Read the model definition and answer for the solid it produces. Units are mm, in the model's axes. A direction names the side the tool comes from. Coordinates: 2 decimals unless noted, no trailing zeros. Loops run counter-clockwise (first coordinate to the right, second up) from the corner with the lowest first, then second, coordinate; pieces in that order, holes last. Notation, with made-up numbers: M 74,-16 L 108,-16 A12 ccw 108,-10 Z; hole C 6,30.5 d6. An arc over 180 degrees is marked long. One line per item, written item: value. Start each with the question number.
1. Determine the mould class of faces 1 (the face through (-34.889, 25, 9)), 2 (the face through (-20.76, 42.07, 0.9)), 3 (the face through (-15, 25, 30.95)) for opening direction X: +X half, -X half, draft (parallel to the pull), parting line (faces both ways), or undercut.
2. The part is cut by section C-C (y = 10.5). Write down the section's boundary in (x, z), then the cut area to 3 significant figures.
3. The part is cut by section B-B (x = -6). Write down the section's boundary in (y, z), then the cut area to 3 significant figures.
4. For faces 4 (the face through (-32.889, 14, 9)), 5 (the face through (-14, 2, 8)), 6 (the face through (-23, 47, 15)), determine the directions among +Z, -Z, +X, -X, +Y, -Y from which every point of the face is accessible in a straight line to the end or side of a thin tool.
5. Flat-ended cylindrical pins translate along their axes: pin 1 (11.5 mm diameter, centred on x = -10, z = 16, fed in from +Y); pin 2 (16 mm diameter, centred on x = -22.5, z = 11, fed in from +Y); pin 3 (2 mm diameter, centred on x = 4.5, z = 14, fed in from -Y). Find the tip coordinate at first contact, or state that the pin passes through.
6. Consider probe 1 along Z at (x, y) = (-24, 10.5); probe 2 along Y at (x, z) = (-31, -1.5); probe 3 along X at (y, z) = (41, -8.5). Determine where each line is inside the solid, lowest interval first.
7. The part is cut by section D-D (y = 45). Write down the section's boundary in (x, z).
8. The part is cut by section A-A (z = 23.5). Write down the section's boundary in (x, y), then the cut area to 3 significant figures.
```python
from build123d import *

# Parameters (mm, degrees)
SKETCH1_W           = 40
SKETCH1_H           = 45
BOSS_EXTRUDE1_DEPTH = 50
SHELL1_T            = -2
SKETCH2_W           = 41
SKETCH2_H           = 15
CUT_EXTRUDE1_DEPTH  = 3
SKETCH4_W           = 41
SKETCH4_H           = 10
BOSS_EXTRUDE2_DEPTH = 20
SKETCH17_R          = 2.5
BOSS_EXTRUDE3_DEPTH = 10
BOSS_EXTRUDE3_TAPER = 3
SKETCH16_R          = 2.5
BOSS_EXTRUDE4_DEPTH = 10
BOSS_EXTRUDE4_TAPER = 3


with BuildPart() as part:
    # Sketch1 → Boss-Extrude1 (new body)
    with BuildSketch(Plane(origin=(0, 0, 0), x_dir=(1, 0, 0), z_dir=(0, 1, 0))):
        with Locations((-14.888700463, -8.449653636)):
            Rectangle(SKETCH1_W, SKETCH1_H)
    extrude(amount=BOSS_EXTRUDE1_DEPTH)

    # Shell1
    shell1_openings = [part.faces().sort_by_distance(p)[0] for p in [
        (-14.888700463, 50, 8.449653636),
    ]]
    offset(amount=SHELL1_T, openings=shell1_openings, kind=Kind.INTERSECTION)

    # Sketch2 → Cut-Extrude1 (cut)
    with BuildSketch(Plane.ZY.offset(-3.111299537)):
        with Locations((8.449653636, 9.5)):
            Rectangle(SKETCH2_W, SKETCH2_H)
    extrude(amount=-CUT_EXTRUDE1_DEPTH, mode=Mode.SUBTRACT)

    # Sketch4 → Boss-Extrude2 (add)
    with BuildSketch(Plane(origin=(-32.888700463, 0, 0), x_dir=(0, 0, -1), z_dir=(1, 0, 0))):
        with Locations((-8.449653636, 32)):
            Rectangle(SKETCH4_W, SKETCH4_H)
    extrude(amount=BOSS_EXTRUDE2_DEPTH)

    # Sketch17 → Boss-Extrude3 (add)
    with BuildSketch(Plane(origin=(0, 37, 0), x_dir=(1, 0, 0), z_dir=(0, 1, 0))):
        with Locations((-22.888700463, -1.572936471)):
            Circle(SKETCH17_R)
    extrude(amount=BOSS_EXTRUDE3_DEPTH, taper=BOSS_EXTRUDE3_TAPER)

    # Sketch16 → Boss-Extrude4 (add)
    with BuildSketch(Plane(origin=(0, 37, 0), x_dir=(1, 0, 0), z_dir=(0, 1, 0))):
        with Locations((-22.81018082, -15.377942678)):
            Circle(SKETCH16_R)
    extrude(amount=BOSS_EXTRUDE4_DEPTH, taper=BOSS_EXTRUDE4_TAPER)


solid = part.part
```
Answer block:
1. face 1: -X half
1. face 2: undercut
1. face 3: draft
2. outline: M -34.89,-14.05 L 5.11,-14.05 L 5.11,-12.05 L -32.89,-12.05 L -32.89,28.95 L 5.11,28.95 L 5.11,30.95 L -34.89,30.95 Z
2. area: 242 mm2
3. outline: M 0,-14.05 L 50,-14.05 L 50,-12.05 L 2,-12.05 L 2,28.95 L 50,28.95 L 50,30.95 L 0,30.95 Z
3. area: 282 mm2
4. face 4: none
4. face 5: +X
4. face 6: +Y
5. pin 1: stops at y = 37
5. pin 2: stops at y = 47
5. pin 3: stops at y = 0
6. probe 1: z = -14.05 to -12.05, 28.95 to 30.95
6. probe 2: y = 0 to 2, 27 to 37
6. probe 3: x = -34.89 to -32.89, 3.11 to 5.11
7. outline: M -34.89,-14.05 L 5.11,-14.05 L 5.11,30.95 L -34.89,30.95 Z; C -22.89,1.57 d4.16; C -22.81,15.38 d4.16; hole M -32.89,-12.05 L 3.11,-12.05 L 3.11,28.95 L -32.89,28.95 Z
8. outline: M -34.89,0 L 5.11,0 L 5.11,2 L -32.89,2 L -32.89,27 L -12.89,27 L -12.89,37 L -32.89,37 L -32.89,50 L -34.89,50 Z; M 3.11,17 L 5.11,17 L 5.11,50 L 3.11,50 Z
8. area: 442 mm2
